```python
from build123d import *
from build123d.topology import SkipClean

# Parameters (mm, degrees)
BOSS_EXTRU_1_DEPTH             = 8
ESQUISSE2_R                    = 2.45
ENL_V_MAT_EXTRU_1_DEPTH        = 3
ENL_V_MAT_EXTRU_2_REACH        = 59.173
ESQUISSE3_R                    = 1.25
ESQUISSE4_R                    = 3
ENL_V_MAT_EXTRU_3_DEPTH        = 2
ENL_V_START                    = -4
ENL_V_MAT_EXTRU_4_DEPTH        = 4
CORPS_D_PLACER_COPIER1_DEPTH   = 8
CORPS_D_PLACER_COPIER1_2_DEPTH = 8
CORPS_D_PLACER_COPIER1_3_DEPTH = 4


# Read off the part's stored shape, not the designer's step: Corps-Déplacer/Copier1
with BuildPart() as part:
    # Esquisse1 → Boss.-Extru.1 (new body)
    with BuildSketch(Plane(origin=(0, 0, 0), x_dir=(1, 0, 0), z_dir=(0, 1, 0))):
        with BuildLine():
            Line((-3, 26.381049961), (-3, 4.963869458))
            ThreePointArc((-3, 4.963869458), (0, -5.8), (3, 4.963869458))
            Line((3, 4.963869458), (3, 38.463869458))
            Line((3, 38.463869458), (-0.867157449, 56.657414832))
            Line((-0.867157449, 56.657414832), (-1.84530505, 56.449503141))
            ThreePointArc((-1.84530505, 56.449503141), (-3.756758837, 55.119060789), (-4.140414176, 52.821988519))
            Line((-4.140414176, 52.821988519), (-3, 49.618950039))
            ThreePointArc((-3, 49.618950039), (0, 38), (-3, 26.381049961))
        make_face()
    extrude(amount=BOSS_EXTRU_1_DEPTH)

    # Esquisse2 → Enlèv. mat.-Extru.1 (cut)
    with BuildSketch(Plane(origin=(0, 8, 0), x_dir=(1, 0, 0), z_dir=(0, 1, 0))):
        with Locations(Location((0, 0, 0), (0, 0, 270))):
            Circle(ESQUISSE2_R)
    extrude(amount=-ENL_V_MAT_EXTRU_1_DEPTH, mode=Mode.SUBTRACT)

    # Esquisse3 → Enlèv. mat.-Extru.2 (cut, up to next)
    with BuildSketch(Plane(origin=(0, 5, 0), x_dir=(1, 0, 0), z_dir=(0, 1, 0)), mode=Mode.PRIVATE) as enl_v_mat_extru_2_sk1:
        with Locations(Location((0, 0, 0), (0, 0, 270))):
            Circle(ESQUISSE3_R)
    enl_v_mat_extru_2_tool1 = extrude(enl_v_mat_extru_2_sk1.sketch, amount=-ENL_V_MAT_EXTRU_2_REACH, mode=Mode.PRIVATE) & part.part
    add(enl_v_mat_extru_2_tool1.solids().sort_by_distance((0, 5, 0))[0], mode=Mode.SUBTRACT)

    # Esquisse4 → Enlèv. mat.-Extru.3 (cut)
    with BuildSketch(Plane.XZ):
        with Locations(Location((0, 0, 0), (0, 0, 270))):
            Circle(ESQUISSE4_R)
    extrude(amount=-ENL_V_MAT_EXTRU_3_DEPTH, mode=Mode.SUBTRACT)

    # Esquisse5 → Enlèv. mat.-Extru.4 (cut)
    with BuildSketch(Plane(origin=(0, 8, 0), x_dir=(1, 0, 0), z_dir=(0, 1, 0)).offset(ENL_V_START)):
        with BuildLine():
            Line((-3, 4.963869458), (-3, 17.24093965))
            ThreePointArc((-3, 17.24093965), (0, 17.5), (3, 17.24093965))
            Line((3, 17.24093965), (3, 4.963869458))
            ThreePointArc((3, 4.963869458), (0, 5.8), (-3, 4.963869458))
        make_face()
    extrude(amount=ENL_V_MAT_EXTRU_4_DEPTH, mode=Mode.SUBTRACT)

    # Corps-Déplacer/Copier1 outline → Corps-Déplacer/Copier1 (cut)
    with SkipClean():  # the faces are left unmerged after this step: merging them gives an invalid solid
        with BuildSketch(Plane(origin=(0, 0, 0), x_dir=(1, 0, 0), z_dir=(0, 1, 0))):
            with BuildLine():
                ThreePointArc((-3, 4.963869458), (0, 5.8), (3, 4.963869458))
                Line((3, 4.963869458), (3, 38.463869458))
                Line((3, 38.463869458), (-0.867157449, 56.657414832))
                Line((-0.867157449, 56.657414832), (-1.84530505, 56.449503141))
                ThreePointArc((-1.84530505, 56.449503141), (-3.756758837, 55.119060789), (-4.140414176, 52.821988519))
                Line((-4.140414176, 52.821988519), (-3, 49.618950039))
                ThreePointArc((-3, 49.618950039), (0, 38), (-3, 26.381049961))
                Line((-3, 26.381049961), (-3, 4.963869458))
            make_face()
        extrude(amount=CORPS_D_PLACER_COPIER1_DEPTH, mode=Mode.SUBTRACT)



with BuildPart() as body_2:
    # Corps-D_placer_Copier1 2 outline → Corps-D_placer_Copier1 2 (new body)
    with BuildSketch(Plane(origin=(0, 0, 0), x_dir=(1, 0, 0), z_dir=(0, 1, 0))):
        with BuildLine():
            Line((3, -38.463869458), (3, -17.24093965))
            ThreePointArc((3, -17.24093965), (0, -17.5), (-3, -17.24093965))
            Line((-3, -17.24093965), (-3, -26.381049961))
            ThreePointArc((-3, -26.381049961), (0, -38), (-3, -49.618950039))
            Line((-3, -49.618950039), (-4.140414176, -52.821988519))
            ThreePointArc((-4.140414176, -52.821988519), (-3.756758837, -55.119060789), (-1.84530505, -56.449503141))
            Line((-1.84530505, -56.449503141), (-0.867157449, -56.657414832))
            Line((-0.867157449, -56.657414832), (3, -38.463869458))
        make_face()
    extrude(amount=CORPS_D_PLACER_COPIER1_2_DEPTH)


with BuildPart() as part_1:
    with SkipClean():  # the faces are left unmerged after this step: merging them gives an invalid solid
        add(part.part)

        add(body_2.part)  # Corps-D_placer_Copier1 3 merges body 2
        # Corps-D_placer_Copier1 3 outline → Corps-D_placer_Copier1 3 (add)
        with BuildSketch(Plane(origin=(0, 0, 0), x_dir=(1, 0, 0), z_dir=(0, 1, 0))):
            with BuildLine():
                Line((3, -17.24093965), (3, -4.963869458))
                ThreePointArc((3, -4.963869458), (0, -5.8), (-3, -4.963869458))
                Line((-3, -4.963869458), (-3, -17.24093965))
                ThreePointArc((-3, -17.24093965), (0, -17.5), (3, -17.24093965))
            make_face()
        extrude(amount=CORPS_D_PLACER_COPIER1_3_DEPTH)


solid = part_1.part
```
Check sheet for the modelled part. Datum: model origin and axes. Units: mm. A direction names the side the tool comes from. Round coordinates to 2 decimals unless told otherwise and drop trailing zeros. Write each loop counter-clockwise with the first axis right and the second up, starting at its lowest first coordinate (ties: lowest second). Pieces come first, ordered by that corner, then holes. Notation, with made-up numbers: (-31, -33.75) -> (-22, -33.75) arc R7 cw to (-22, -22.75) -> close; hole circle Ø10 at (-20, 64.25). An arc over 180 degrees is marked (long way). Put each result on its own line as item: value.
(1) Sectioned sample at A-A (y = 7). Enter the section's corners in (x, z).
Values found:
outline: circle Ø11.6 at (0, 0); (-4.14, 52.82) -> (-3, 49.62) arc R24 cw to (-3, 26.38) -> (-3, 17.24) arc R17.5 cw to (3, 17.24) -> (3, 38.46) -> (-0.87, 56.66) -> (-1.85, 56.45) arc R3 ccw to start; hole circle Ø4.9 at (0, 0)
(2) Material ranges on line 1 (X direction, y = 0.8, z = 0); line 2 (X direction, y = 3.6, z = 0); line 3 (X direction, y = 3.25, z = 16.5), recorded low to high.
Values found:
line 1: x = -5.8 to -3, 3 to 5.8
line 2: x = -5.8 to -1.25, 1.25 to 5.8
line 3: x = -3 to 3
(3) Tool access check on faces 1 (the face through (0, 6, 17.5)), 2 (the face through (0.9, 0.99, -2.86)), 3 (the face through (3, 4, 26)), 4 (the face through (-3, 3, 18)). Record the directions out of +Z, -Z, +X, -X, +Y, -Y that give a thin tool (end or side, any length) a straight path to the whole face; none if there is none.
Values found:
face 1: +Y
face 2: -Y
face 3: +Z, +X, +Y, -Y
face 4: -X, +Y, -Y
(4) Sectioned sample at C-C (y = 3). Enter the section's corners in (x, z), plus the area to 3 significant figures.
Values found:
outline: (-4.14, 52.82) -> (-3, 49.62) arc R24 cw to (-3, 26.38) -> (-3, 4.96) arc R5.8 ccw (long way) to (3, 4.96) -> (3, 38.46) -> (-0.87, 56.66) -> (-1.85, 56.45) arc R3 ccw to start; hole circle Ø2.5 at (0, 0)
area: 329 mm^2
(5) Sectioned sample at D-D (z = 19.5). Enter the section's corners in (x, y), plus the area to 3 significant figures.
Values found:
outline: (-3, 0) -> (3, 0) -> (3, 8) -> (-3, 8) -> close
area: 48.0 mm^2
(6) Sectioned sample at B-B (z = 0). Enter the section's corners in (x, y).
Values found:
outline: (-5.8, 0) -> (-3, 0) -> (-3, 2) -> (-1.25, 2) -> (-1.25, 5) -> (-2.45, 5) -> (-2.45, 8) -> (-5.8, 8) -> close; (1.25, 2) -> (3, 2) -> (3, 0) -> (5.8, 0) -> (5.8, 8) -> (2.45, 8) -> (2.45, 5) -> (1.25, 5) -> close
(7) Mould release check, pull along X, two halves, no side actions. Record for faces 5 (the face through (0.736, 6.521, 2.337)), 6 (the face through (0, 0, 18)), 7 (the face through (1.04, 3.94, 47.69)), 8 (the face through (-1.363, 3.944, 56.552)): released by +X, released by -X, zero draft, split by the parting line, or undercut.
Values found:
face 5: undercut
face 6: zero draft
face 7: released by +X
face 8: released by -X
(8) Go/stop test with flat-tipped pins: pin 1 Ø3 at (x, z) = (1.5, 13) entering from +Y; pin 2 Ø2 at (x, z) = (3, 44) entering from -Y; pin 3 Ø2 at (x, y) = (-4, 7) entering from -Z; pin 4 Ø1.5 at (x, z) = (0, 1) entering from +Y. Record where each tip stops, or that it passes through.
Values found:
pin 1: stops at y = 4
pin 2: passes through
pin 3: stops at z = -4.96
pin 4: stops at y = 5
